from build123d import *

# Parameters (mm, degrees)
CROQUIS1_R              = 26.5
SALIENTE_EXTRUIR1_DEPTH = 5
SALIENTE_EXTRUIR2_DEPTH = 4
CROQUIS3_R              = 5
SALIENTE_EXTRUIR3_DEPTH = 4
CROQUIS4_R              = 2.5
CORTAR_EXTRUIR1_DEPTH   = 2
CROQUIS5_R              = 1.5
CORTAR_EXTRUIR2_DEPTH   = 49.769867746
MATRIZC1_COUNT          = 4
CROQUIS6_R              = 1
CORTAR_EXTRUIR3_DEPTH   = 58.493477891


with BuildPart() as part:
    # Croquis1 → Saliente-Extruir1 (new body)
    with BuildSketch(Plane(origin=(0, 0, 0), x_dir=(1, 0, 0), z_dir=(0, 1, 0))):
        with Locations(Location((0, 0, 0), (0, 0, 270))):
            Circle(CROQUIS1_R)
    extrude(amount=SALIENTE_EXTRUIR1_DEPTH)

    # Croquis2 → Saliente-Extruir2 (add)
    with BuildSketch(Plane(origin=(0, 0, 0), x_dir=(1, 0, 0), z_dir=(0, 1, 0))):
        with BuildLine():
            Line((-5.029139679, 25.088960855), (-2.702516138, 31.293290297))
            ThreePointArc((-2.702516138, 31.293290297), (0, 40.5), (2.702516138, 31.293290297))
            Line((2.702516138, 31.293290297), (5.029139679, 25.088960855))
            Line((5.029139679, 25.088960855), (-5.029139679, 25.088960855))
        make_face()
    saliente_extruir2 = extrude(amount=SALIENTE_EXTRUIR2_DEPTH)

    # Croquis3 → Saliente-Extruir3 (add)
    with BuildSketch(Plane(origin=(0, 4, 0), x_dir=(1, 0, 0), z_dir=(0, 1, 0))):
        with Locations(Location((0, 35.5, 0), (0, 0, 237.282097692))):
            Circle(CROQUIS3_R)
    saliente_extruir3 = extrude(amount=SALIENTE_EXTRUIR3_DEPTH)

    # Croquis4 → Cortar-Extruir1 (cut)
    with BuildSketch(Plane(origin=(0, 8, 0), x_dir=(1, 0, 0), z_dir=(0, 1, 0))):
        with Locations(Location((0, 35.5, 0), (0, 0, 270))):
            Circle(CROQUIS4_R)
    cortar_extruir1 = extrude(amount=-CORTAR_EXTRUIR1_DEPTH, mode=Mode.SUBTRACT)

    # Croquis5 → Cortar-Extruir2 (cut, through all)
    with BuildSketch(Plane(origin=(0, 6, 0), x_dir=(1, 0, 0), z_dir=(0, 1, 0))):
        with Locations(Location((0, 35.5, 0), (0, 0, 270))):
            Circle(CROQUIS5_R)
    cortar_extruir2 = extrude(amount=-CORTAR_EXTRUIR2_DEPTH, mode=Mode.SUBTRACT)

    # MatrizC1: Saliente-Extruir2, Saliente-Extruir3, Cortar-Extruir1, Cortar-Extruir2 ×4 about axis
    matrizc1_axis = Axis((0, 0, 0), (0, 1, 0))
    add([saliente_extruir2.rotate(matrizc1_axis, i * 360 / MATRIZC1_COUNT) for i in range(1, MATRIZC1_COUNT)])
    add([saliente_extruir3.rotate(matrizc1_axis, i * 360 / MATRIZC1_COUNT) for i in range(1, MATRIZC1_COUNT)])
    add([cortar_extruir1.rotate(matrizc1_axis, i * 360 / MATRIZC1_COUNT) for i in range(1, MATRIZC1_COUNT)], mode=Mode.SUBTRACT)
    add([cortar_extruir2.rotate(matrizc1_axis, i * 360 / MATRIZC1_COUNT) for i in range(1, MATRIZC1_COUNT)], mode=Mode.SUBTRACT)

    # Croquis6 → Cortar-Extruir3 (cut, through all)
    with BuildSketch(Plane(origin=(0, 5, 0), x_dir=(1, 0, 0), z_dir=(0, 1, 0))):
        with Locations(Location((-4.949747468, 4.949747468, 0), (0, 0, 270))):
            Circle(CROQUIS6_R)
        with Locations(Location((4.949747468, -4.949747468, 0), (0, 0, 270))):
            Circle(CROQUIS6_R)
    extrude(amount=-CORTAR_EXTRUIR3_DEPTH, mode=Mode.SUBTRACT)


solid = part.part
Geometry check sheet. Reference: the model listing, model coordinates, mm. A direction names the side the tool comes from. Give positions to 0.01 mm unless a question says otherwise; leave off trailing zeros. Loops run counter-clockwise (first coordinate to the right, second up) from the corner with the lowest first, then second, coordinate; pieces in that order, holes last. Notation, with made-up numbers: M 78.25,65 L 123.25,65 A20 ccw 123.25,79 Z; hole C 13.5,-36.5 d3. An arc over 180 degrees is marked long. Write each question's results on one line, items separated by ' | '.
1) Tool access check on faces 5 (the face through (5.94, 2.54, 4.82)), 6 (the face through (34, 6, -1)), 7 (the face through (3.692, 1.972, 28.654)). Record the directions out of +Z, -Z, +X, -X, +Y, -Y that give a thin tool (end or side, any length) a straight path to the whole face; none if there is none.
Answers follow:
face 5: +Y, -Y | face 6: +Y | face 7: +X, +Y, -Y
2) Release check for a two-part mould opening along X. For faces 1 (the face through (28.727, 1.972, 3.665)), 2 (the face through (0, 4, -28)), 3 (the face through (-36.7, 3, 0.9)), 4 (the face through (3.665, 1.972, -28.727)) record: +X half, -X half, draft (parallel to the pull), parting line (faces both ways), or undercut.
Answers follow:
face 1: undercut | face 2: draft | face 3: undercut | face 4: +X half
3) Section check B-B, the plane x = 0. Record the boundary of the cut face in (y, z).
Answers follow:
outline: M 0,-40.5 L 8,-40.5 L 8,-38 L 6,-38 L 6,-37 L 0,-37 Z; M 0,-34 L 6,-34 L 6,-33 L 8,-33 L 8,-30.5 L 4,-30.5 L 4,-26.5 L 5,-26.5 L 5,26.5 L 4,26.5 L 4,30.5 L 8,30.5 L 8,33 L 6,33 L 6,34 L 0,34 Z; M 0,37 L 6,37 L 6,38 L 8,38 L 8,40.5 L 0,40.5 Z
4) Gauge pin test, flat ends, axial feed: pin 1 (2 mm diameter, centred on x = -7, y = 3, fed in from +Z); pin 2 (1.8 mm diameter, centred on x = 0, z = -35.5, fed in from -Y) (1 decimal); pin 3 (1.6 mm diameter, centred on x = 28, z = 2, fed in from +Y); pin 4 (1.5 mm diameter, centred on x = 36.5, z = -0.5, fed in from +Y). Record the tip position at first contact, or that the pin passes through.
Answers follow:
pin 1: z = 25.81 | pin 2: through | pin 3: y = 4 | pin 4: y = 6
5) Section check D-D, the plane x = 35.5. Record the boundary of the cut face in (y, z), plus the area to 3 significant figures.
Answers follow:
outline: M 0,-5 L 8,-5 L 8,-2.5 L 6,-2.5 L 6,-1.5 L 0,-1.5 Z; M 0,1.5 L 6,1.5 L 6,2.5 L 8,2.5 L 8,5 L 0,5 Z | area: 52.0 mm2
6) Thickness scan on line 1 (X direction, y = 4.1, z = -35.5); line 2 (Z direction, x = -35.5, y = 7). Record the ranges inside material, lowest first.
Answers follow:
line 1: -5 to -1.5, 1.5 to 5 | line 2: -5 to -2.5, 2.5 to 5
7) Section check C-C, the plane z = 0. Record the boundary of the cut face in (x, y).
Answers follow:
outline: M -40.5,0 L -37,0 L -37,6 L -38,6 L -38,8 L -40.5,8 Z; M -34,0 L 34,0 L 34,6 L 33,6 L 33,8 L 30.5,8 L 30.5,4 L 26.5,4 L 26.5,5 L -26.5,5 L -26.5,4 L -30.5,4 L -30.5,8 L -33,8 L -33,6 L -34,6 Z; M 37,0 L 40.5,0 L 40.5,8 L 38,8 L 38,6 L 37,6 Z
8) Section check A-A, the plane z = 35.5. Record the boundary of the cut face in (x, y).
Answers follow:
outline: M -5,0 L -1.5,0 L -1.5,6 L -2.5,6 L -2.5,8 L -5,8 Z; M 1.5,0 L 5,0 L 5,8 L 2.5,8 L 2.5,6 L 1.5,6 Z
